Geometry: final body of the model. Coordinates: model frame, mm. A direction names the side the tool comes from. Coordinates: 2 decimals unless noted, no trailing zeros. Loops run counter-clockwise (first coordinate to the right, second up) from the corner with the lowest first, then second, coordinate; pieces in that order, holes last. Notation, with made-up numbers: (12, 66) - (21, 66) arc R10 ccw to (21, 80) - close; hole circle Ø10 at (54, -38). An arc over 180 degrees is marked (long way). Answer in a Markdown table with one row per item.
from build123d import *

# Parameters (mm, degrees)
F0_W     = 63.5
F0_H     = 25.4
F1_DEPTH = 31.75
F3_DEPTH = 25.4


with BuildPart() as f1:
    # F0 (on Top) → F1 (new body)
    with BuildSketch(Plane.XY):
        with Locations((-31.75, 12.7)):
            Rectangle(F0_W, F0_H)
    extrude(amount=F1_DEPTH)

    # F2 (on face) → F3 (cut)
    with BuildSketch(Plane(origin=(0, 0, 0), x_dir=(1, 0, 0), z_dir=(0, 0, -1))):
        with BuildLine():
            ThreePointArc((-50.984073, 0), (-42.817071, -9.834289), (-30.535549, -13.380745))
            ThreePointArc((-30.535549, -13.380745), (-19.265496, -9.823114), (-12.694554, 0))
            Line((-12.694554, 0), (-50.984073, 0))
        make_face()
    extrude(amount=-F3_DEPTH, mode=Mode.SUBTRACT)


solid = f1.part
(1) Ray query, probe 1 along Y at (x, z) = (-30.5, 21); probe 2 along Z at (x, y) = (-47, 3); probe 3 along X at (y, z) = (6.5, 10). Return the intervals inside material, ascending.
Verdict:
| item | result |
|---|---|
| probe 1 | y = 13.38 to 25.4 |
| probe 2 | z = 25.4 to 31.75 |
| probe 3 | x = -63.5 to -46.78, -15.88 to 0 |
(2) Cut plane A-A on y = 3.75. Output: boundary loops of the cut face in (x, z), then the cut area to 3 significant figures.
Verdict:
| item | result |
|---|---|
| outline | (-63.5, 0) - (-48.97, 0) - (-48.97, 25.4) - (-14.13, 25.4) - (-14.13, 0) - (0, 0) - (0, 31.75) - (-63.5, 31.75) - close |
| area | 1,130 mm² |
(3) Cut plane D-D on y = 9. Output: boundary loops of the cut face in (x, z), then the cut area to 3 significant figures.
Verdict:
| item | result |
|---|---|
| outline | (-63.5, 0) - (-44, 0) - (-44, 25.4) - (-18.25, 25.4) - (-18.25, 0) - (0, 0) - (0, 31.75) - (-63.5, 31.75) - close |
| area | 1,360 mm² |
(4) Access query for faces 1 (the face through (-32, 13, 31.75)), 2 (the face through (-42.969, 9.734, 12.522)). Directions: +Z, -Z, +X, -X, +Y, -Y. A direction counts if a zero-diameter tool reaches every point of the face in a straight line with its end or side. Return the directions, or none.
Verdict:
| item | result |
|---|---|
| face 1 | +Z, +X, -X, +Y, -Y |
| face 2 | -Z, -Y |
(5) Cut plane B-B on z = 5.5. Output: boundary loops of the cut face in (x, y), then the cut area to 3 significant figures.
Verdict:
| item | result |
|---|---|
| outline | (-63.5, 0) - (-50.98, 0) arc R21.75 cw to (-30.54, 13.38) arc R17.83 cw to (-12.69, 0) - (0, 0) - (0, 25.4) - (-63.5, 25.4) - close |
| area | 1,230 mm² |
(6) First-contact query: pin 1 Ø6 at (x, z) = (-28.5, 19.5) entering from -Y; pin 2 Ø3 at (x, z) = (-31.5, 19.5) entering from -Y. Flat tips, straight axial feed; report the tip coordinate or a pass-through.
Verdict:
| item | result |
|---|---|
| pin 1 | stops at y = 12.82 |
| pin 2 | stops at y = 13.28 |
(7) Cut plane C-C on x = -34. Output: boundary loops of the cut face in (y, z).
Verdict:
| item | result |
|---|---|
| outline | (0, 25.4) - (13.16, 25.4) - (13.16, 0) - (25.4, 0) - (25.4, 31.75) - (0, 31.75) - close |
